from build123d import *

# Parameters (mm, degrees)
BOSS_EXTRUDE1_DEPTH = 2
BOSS_EXTRUDE2_DEPTH = 2
BOSS_EXTRUDE2_TAPER = 45
BOSS_EXTRUDE3_DEPTH = 5
BOSS_EXTRUDE4_START = 1
BOSS_EXTRUDE4_DEPTH = 1
CHAMFER1_SIZE       = 1
SKETCH6_R           = 2.5
CUT_EXTRUDE1_DEPTH  = 55.939106152
SKETCH8_R           = 2.5
CUT_EXTRUDE2_DEPTH  = 55.694698419
BOSS_EXTRUDE5_DEPTH = 10
FILLET1_R           = 5
SKETCH10_W          = 6
SKETCH10_H          = 3
CUT_EXTRUDE3_DEPTH  = 9
CUT_EXTRUDE4_REACH  = 56.695
SKETCH11_R          = 1.7


# Some blends are built 0.0001 mm under size
with BuildPart() as part:
    # Sketch1 → Boss-Extrude1 (new body)
    with BuildSketch(Plane(origin=(0, 0, 0), x_dir=(0, 0, -1), z_dir=(1, 0, 0))):
        with BuildLine():
            Line((0, 0), (35, 0))
            Line((35, 0), (35, 8.213))
            ThreePointArc((35, 8.213), (34.84410791, 9.971846057), (34.381292109, 11.675854077))
            Line((34.381292109, 11.675854077), (26.150489454, 33.974097745))
            ThreePointArc((26.150489454, 33.974097745), (17.499798515, 40.001999998), (8.849371011, 33.973719703))
            Line((8.849371011, 33.973719703), (0.618556568, 11.672444098))
            ThreePointArc((0.618556568, 11.672444098), (0.15585366, 9.968630956), (0, 8.21))
            Line((0, 8.21), (0, 0))
        make_face()
    extrude(amount=BOSS_EXTRUDE1_DEPTH)

    # Sketch2 → Boss-Extrude2 (add)
    with BuildSketch(Plane(origin=(2, 0, 0), x_dir=(0, 0, -1), z_dir=(1, 0, 0))):
        with BuildLine():
            Line((8.849371011, 33.973719703), (0.618556568, 11.672444098))
            ThreePointArc((0.618556568, 11.672444098), (0.15585366, 9.968630956), (0, 8.21))
            Line((0, 8.21), (0, 0))
            Line((0, 0), (35, 0))
            Line((35, 0), (35, 8.213))
            ThreePointArc((35, 8.213), (34.84410791, 9.971846057), (34.381292109, 11.675854077))
            Line((34.381292109, 11.675854077), (26.150489454, 33.974097745))
            ThreePointArc((26.150489454, 33.974097745), (17.499798515, 40.001999998), (8.849371011, 33.973719703))
        make_face()
    extrude(amount=BOSS_EXTRUDE2_DEPTH, taper=BOSS_EXTRUDE2_TAPER)

    # Sketch4 → Boss-Extrude3 (add)
    with BuildSketch(Plane.XZ):
        with BuildLine():
            Line((0, 0), (2, 0))
            ThreePointArc((2, 0), (12.897674733, -17.5), (2, -35))
            Line((2, -35), (0, -35))
            Line((0, -35), (0, 0))
        make_face()
    extrude(amount=-BOSS_EXTRUDE3_DEPTH)

    # Sketch5 → Boss-Extrude4 (add)
    with BuildSketch(Plane.ZY.offset(BOSS_EXTRUDE4_START)):
        with BuildLine():
            Line((0, 5.5), (0, 8.21))
            ThreePointArc((0, 8.21), (-0.15585366, 9.968630956), (-0.618556568, 11.672444098))
            Line((-0.618556568, 11.672444098), (-1.662133105, 14.5))
            Line((-1.662133105, 14.5), (-33.338833873, 14.5))
            Line((-33.338833873, 14.5), (-34.381292109, 11.675854077))
            ThreePointArc((-34.381292109, 11.675854077), (-34.84410791, 9.971846057), (-35, 8.213))
            Line((-35, 8.213), (-35, 5.5))
            Line((-35, 5.5), (0, 5.5))
        make_face()
    extrude(amount=-BOSS_EXTRUDE4_DEPTH)

    # Chamfer1
    chamfer1_edges = [part.edges().sort_by_distance(p)[0] for p in [
        (-1, 14.5, -17.500483489),
        (-1, 5.5, -17.5),
    ]]
    chamfer(chamfer1_edges, length=CHAMFER1_SIZE - 0.0001)  # a hair under: the kernel refuses the full size

    # Chamfer2
    # the kernel refuses this chamfer: 1 mm, written as the material it takes off along each edge
    with BuildSketch(Plane(origin=(-1, 0.327860829, 0), x_dir=(-0.027495876610586275, 0, -0.9996219169112968), z_dir=(0, 1, 0))) as chamfer2_piece_1:
        with BuildLine():
            Line((1.028673195, 0), (-0.056547155, -1.027117794))
            Line((-0.056547155, -1.027117794), (-0.076539593, -1.026567876))
            ThreePointArc((-0.076539593, -1.026567876), (-0.034129227, -0.51339783), (-0.019992438, 0.000549918))
            Line((-0.019992438, 0.000549918), (0.000549918, 0.019992438))
            ThreePointArc((0.000549918, 0.019992438), (0.514497665, 0.00585565), (1.029223113, 0.019992438))
            Line((1.029223113, 0.019992438), (1.028673195, 0))
        make_face()
    extrude(amount=14.054178342, mode=Mode.SUBTRACT)
    with BuildSketch(Plane(origin=(-1, 14.385039171, -35), x_dir=(-0.0274958766105862, 0, 0.9996219169112968), z_dir=(0, -1, 0))) as chamfer2_piece_2:
        with BuildLine():
            Line((1.028673195, 0), (-0.056547155, -1.027117794))
            Line((-0.056547155, -1.027117794), (-0.076539593, -1.026567876))
            ThreePointArc((-0.076539593, -1.026567876), (-0.034129227, -0.51339783), (-0.019992438, 0.000549918))
            Line((-0.019992438, 0.000549918), (0.000549918, 0.019992438))
            ThreePointArc((0.000549918, 0.019992438), (0.514497665, 0.00585565), (1.029223113, 0.019992438))
            Line((1.029223113, 0.019992438), (1.028673195, 0))
        make_face()
    extrude(amount=14.057178342, mode=Mode.SUBTRACT)

    # Sketch6 → Cut-Extrude1 (cut, through all)
    with BuildSketch(Plane.ZY.offset(1)):
        with Locations((-27.5, 10)):
            Circle(SKETCH6_R)
        with Locations((-7.5, 10)):
            Circle(SKETCH6_R)
    extrude(amount=-CUT_EXTRUDE1_DEPTH, mode=Mode.SUBTRACT)

    # Sketch8 → Cut-Extrude2 (cut, through all)
    with BuildSketch(Plane.ZY):
        with Locations((-17.5, 29.999)):
            Circle(SKETCH8_R)
    extrude(amount=-CUT_EXTRUDE2_DEPTH, mode=Mode.SUBTRACT)

    # Sketch9 → Boss-Extrude5 (add)
    with BuildSketch(Plane(origin=(0, 0, -22.5), x_dir=(-1, 0, 0), z_dir=(0, 0, -1))):
        Polygon((-4, 5), (-4, 25), (-10, 5), align=None)
    extrude(amount=-BOSS_EXTRUDE5_DEPTH)

    # Fillet1
    fillet1_edges = [part.edges().sort_by_distance(p)[0] for p in [
        (7, 5, -12.5),
        (7, 5, -22.5),
    ]]
    fillet(fillet1_edges, radius=FILLET1_R)

    # Sketch10 → Cut-Extrude3 (cut)
    with BuildSketch(Plane.ZY):
        with Locations((-17.5, 3.5)):
            Rectangle(SKETCH10_W, SKETCH10_H)
    extrude(amount=-CUT_EXTRUDE3_DEPTH, mode=Mode.SUBTRACT)

    # Sketch11 → Cut-Extrude4 (cut, up to next)
    with BuildSketch(Plane.XZ, mode=Mode.PRIVATE) as cut_extrude4_sk1:
        with Locations(Location((5, -17.5, 0), (0, 0, 270))):
            Circle(SKETCH11_R)
    cut_extrude4_tool1 = extrude(cut_extrude4_sk1.sketch, amount=-CUT_EXTRUDE4_REACH, mode=Mode.PRIVATE) & part.part
    add(cut_extrude4_tool1.solids().sort_by_distance((5, 0, -17.5))[0], mode=Mode.SUBTRACT)


solid = part.part
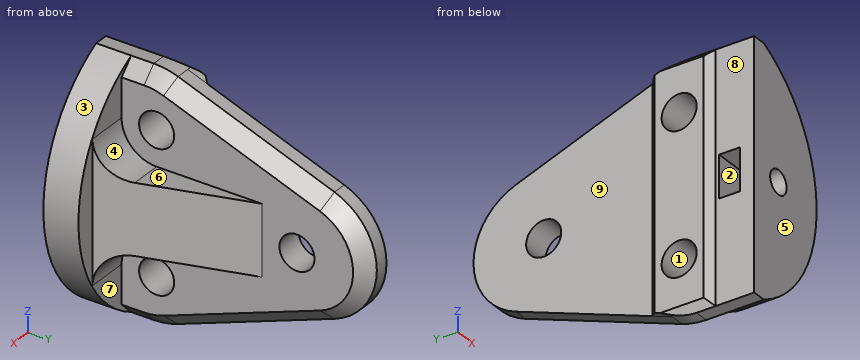
CAD build for the part. Positions are in the model's coordinates, mm. Face numbers are marked on the shaded views. A direction names the side the tool comes from. Round coordinates to 2 decimals unless told otherwise and drop trailing zeros. Write each loop counter-clockwise with the first axis right and the second up, starting at its lowest first coordinate (ties: lowest second). Pieces come first, ordered by that corner, then holes.
(1) Slice it at A-A, the plane y = 4. Write the cut outline in (x, z).
(2) Drop flat-ended pins along their axis: P1, Ø1.3, axis at x = 6.5, y = 15, coming from the +Z side; P2, Ø4.5, axis at y = 3, z = -16.5, coming from the -X side; P3, Ø0.9, axis at y = 3, z = -18, coming from the -X side; P4, Ø4, axis at y = 10, z = -27.5, coming from the +X side. Give the stop position or say it passes through.
(3) Probe line 1 along Z through (x, y) = (0, 8); line 2 along X through (y, z) = (1.3, -17.5); line 3 along Z through (x, y) = (5.5, 11). List the from-to ranges inside material, lowest first.
(4) Slice it at D-D, the plane x = 5. Write the cut outline in (y, z), and give its area (3 significant figures).
(5) Slice it at C-C, the plane z = -17.5. Count the separate pieces of the cut face and the enclosed holes in it, and give its area (3 significant figures).
(6) 3-axis set-ups, long thin cutter, end or side, ignore diameter. For the marked faces 5, 6, 7, 8 and 9: which of +Z, -Z, +X, -X, +Y, -Y reach the whole face in a straight line?
(7) Slice it at B-B, the plane x = 1.25. Write the cut outline in (y, z), and give its area (3 significant figures).
(8) Mould opens along Y. For the marked faces 1, 2, 3 and 4 say: pulls with the +Y half, pulls with the -Y half, needs draft (parallel to the pull), parting line crosses it, or undercut.
From the geometry:
1. outline: (0, -35) - (2, -35) arc R19.5 ccw to (2, 0) - (0, 0) - (0, -14.5) - (9, -14.5) - (9, -20.5) - (0, -20.5) - close
2. P1: stops at z = -12.5
2. P2: stops at x = 0
2. P3: stops at x = 9
2. P4: passes through
3. line 1: z = -35 to -29, -26 to -9, -6 to 0
3. line 2: x = 0 to 3.3, 6.7 to 12.9
3. line 3: z = -22.5 to -12.5
4. outline: (0, -33.17) - (5, -33.17) - (5, -27.5) arc R5 cw to (10, -22.5) - (21.67, -22.5) - (21.67, -12.5) - (10, -12.5) arc R5 cw to (5, -7.5) - (5, -1.83) - (0, -1.83) - (0, -15.8) - (2, -15.8) - (2, -14.5) - (5, -14.5) - (5, -20.5) - (2, -20.5) - (2, -19.2) - (0, -19.2) - close
4. area: 309 mm2
5. separate pieces: 3
5. enclosed holes: 0
5. area: 217 mm2
6. face 5: +Z, -Z, +X, -X, -Y
6. face 6: +Z, +X, +Y
6. face 7: +X, +Y
6. face 8: +Z, -Z, -X, -Y
6. face 9: +Z, -Z, -X, +Y
7. outline: (0, -35) - (8.21, -35) arc R10 ccw to (11.68, -34.38) - (33.97, -26.15) arc R9.22 ccw to (33.97, -8.85) - (11.67, -0.62) arc R10 ccw to (8.21, 0) - (0, 0) - close; hole (2, -20.5) - (5, -20.5) - (5, -14.5) - (2, -14.5) - close; hole circle Ø5 at (10, -27.5); hole circle Ø5 at (10, -7.5); hole circle Ø5 at (30, -17.5)
7. area: 976 mm2
8. face 1: undercut
8. face 2: undercut
8. face 3: needs draft
8. face 4: pulls with the +Y half
